```python
from build123d import *

# Parameters (mm, degrees)
EXTRUDE_1_DEPTH          = 7.5
CUT_EXTRUDE_1_DEPTH      = 30.546573405
CUT_EXTRUDE_1_DEPTH_BACK = 30.546573405
SKETCH_2_W               = 20
SKETCH_2_H               = 20
SKETCH_11_W              = 29.504788154
SKETCH_11_H              = 47.493911142
CUT_EXTRUDE_7_DEPTH      = 1
SKETCH_12_W              = 20.237973212
SKETCH_12_H              = 25.719397838
CUT_EXTRUDE_8_DEPTH      = 1
FILLET_1_R               = 5
FILLET_2_R               = 5
CUT_EXTRUDE_2_DEPTH      = 39.745967532
CUT_EXTRUDE_2_DEPTH_BACK = 39.745967532
SKETCH_3_R               = 4.2
CUT_EXTRUDE_3_DEPTH      = 39.745967532
CUT_EXTRUDE_3_DEPTH_BACK = 39.745967532
SKETCH_4_R               = 4.2
EXTRUDE_2_DEPTH          = 15
SKETCH_6_R               = 4.2
SKETCH_6_R_2             = 3.5
EXTRUDE_3_DEPTH          = 3.4
EXTRUDE_START            = -3.4
SKETCH_13_R              = 4.2
SKETCH_13_R_2            = 3.5
EXTRUDE_4_DEPTH          = 3.4
SKETCH_14_R              = 50
EXTRUDE_5_DEPTH          = 10
CUT_EXTRUDE_START        = -10
CUT_EXTRUDE_9_DEPTH      = 10
CHAMFER_1_SIZE           = 5
CUT_EXTRUDE_10_DEPTH     = 15
PATTERN_CIRCULAR_1_COUNT = 4


with BuildPart() as part:
    # ｽｹｯﾁ1 → ﾎﾞｽ - 押し出し1 (new, symmetric)
    with BuildSketch(Plane.XY):
        Polygon((7.455844123, -18), (18, -7.455844123), (18, 7.455844123), (7.455844123, 18), (-7.455844123, 18), (-18, 7.455844123), (-18, -7.455844123), (-7.455844123, -18), align=None)
    extrude(amount=EXTRUDE_1_DEPTH, both=True)

    # ｽｹｯﾁ2 → ｶｯﾄ - 押し出し1 (cut, two sides: drawn at the far end of the back side and taken through both)
    with BuildSketch(Plane.XY.offset(7.5).offset(-CUT_EXTRUDE_1_DEPTH_BACK)):
        Rectangle(SKETCH_2_W, SKETCH_2_H)
    extrude(amount=CUT_EXTRUDE_1_DEPTH + CUT_EXTRUDE_1_DEPTH_BACK, mode=Mode.SUBTRACT)

    # ｽｹｯﾁ11 → ｶｯﾄ - 押し出し7 (cut)
    with BuildSketch(Plane(origin=(0, 18, 0), x_dir=(1, 0, 0), z_dir=(0, 1, 0))):
        Rectangle(SKETCH_11_W, SKETCH_11_H)
    cut_extrude_7 = extrude(amount=-CUT_EXTRUDE_7_DEPTH, mode=Mode.SUBTRACT)

    # ﾐﾗｰ1: ｶｯﾄ - 押し出し7 across plane
    add(cut_extrude_7.mirror(Plane.ZX), mode=Mode.SUBTRACT)

    # ｽｹｯﾁ12 → ｶｯﾄ - 押し出し8 (cut)
    with BuildSketch(Plane.ZY.offset(18)):
        Rectangle(SKETCH_12_W, SKETCH_12_H)
    cut_extrude_8 = extrude(amount=-CUT_EXTRUDE_8_DEPTH, mode=Mode.SUBTRACT)

    # ﾐﾗｰ2: ｶｯﾄ - 押し出し8 across plane
    add(cut_extrude_8.mirror(Plane(origin=(0, 0, 0), x_dir=(0, 0, 1), z_dir=(1, 0, 0))), mode=Mode.SUBTRACT)

    # ﾌｨﾚｯﾄ1
    fillet_1_edges = [part.edges().sort_by_distance(p)[0] for p in [
        (-10, -10, 0),
        (-10, 10, 0),
        (10, 10, 0),
        (10, -10, 0),
    ]]
    fillet(fillet_1_edges, radius=FILLET_1_R)

    # ﾌｨﾚｯﾄ2
    fillet_2_edges = [part.edges().sort_by_distance(p)[0] for p in [
        (17, 8.455844123, 0),
        (17, -8.455844123, 0),
        (-8.455844123, 17, 0),
        (8.455844123, 17, 0),
        (8.455844123, -17, 0),
        (-8.455844123, -17, 0),
        (-17, -8.455844123, 0),
        (-17, 8.455844123, 0),
    ]]
    fillet(fillet_2_edges, radius=FILLET_2_R)

    # ｽｹｯﾁ3 → ｶｯﾄ - 押し出し2 (cut, two sides: drawn at the far end of the back side and taken through both)
    with BuildSketch(Plane.XZ.offset(17).offset(-CUT_EXTRUDE_2_DEPTH_BACK)):
        with Locations(Location((0, 0, 0), (0, 0, 270))):
            Circle(SKETCH_3_R)
    extrude(amount=CUT_EXTRUDE_2_DEPTH + CUT_EXTRUDE_2_DEPTH_BACK, mode=Mode.SUBTRACT)

    # ｽｹｯﾁ4 → ｶｯﾄ - 押し出し3 (cut, two sides: drawn at the far end of the back side and taken through both)
    with BuildSketch(Plane(origin=(17, 0, 0), x_dir=(0, 0, -1), z_dir=(1, 0, 0)).offset(-CUT_EXTRUDE_3_DEPTH_BACK)):
        Circle(SKETCH_4_R)
    extrude(amount=CUT_EXTRUDE_3_DEPTH + CUT_EXTRUDE_3_DEPTH_BACK, mode=Mode.SUBTRACT)

    # ｽｹｯﾁ5 → ﾎﾞｽ - 押し出し2 (add)
    with BuildSketch(Plane.XY.offset(7.5)):
        with BuildLine():
            Line((17, -6.384776311), (17, 6.384776311))
            ThreePointArc((17, 6.384776311), (16.619397663, 8.298193473), (15.535533906, 9.920310217))
            Line((15.535533906, 9.920310217), (9.920310217, 15.535533906))
            ThreePointArc((9.920310217, 15.535533906), (8.298193473, 16.619397663), (6.384776311, 17))
            Line((6.384776311, 17), (-6.384776311, 17))
            ThreePointArc((-6.384776311, 17), (-8.298193473, 16.619397663), (-9.920310217, 15.535533906))
            Line((-9.920310217, 15.535533906), (-15.535533906, 9.920310217))
            ThreePointArc((-15.535533906, 9.920310217), (-16.619397663, 8.298193473), (-17, 6.384776311))
            Line((-17, 6.384776311), (-17, -6.384776311))
            ThreePointArc((-17, -6.384776311), (-16.619397663, -8.298193473), (-15.535533906, -9.920310217))
            Line((-15.535533906, -9.920310217), (-9.920310217, -15.535533906))
            ThreePointArc((-9.920310217, -15.535533906), (-8.298193473, -16.619397663), (-6.384776311, -17))
            Line((-6.384776311, -17), (6.384776311, -17))
            ThreePointArc((6.384776311, -17), (8.298193473, -16.619397663), (9.920310217, -15.535533906))
            Line((9.920310217, -15.535533906), (15.535533906, -9.920310217))
            ThreePointArc((15.535533906, -9.920310217), (16.619397663, -8.298193473), (17, -6.384776311))
        make_face()
        with BuildLine():
            Line((5, 10), (-5, 10))
            ThreePointArc((-5, 10), (-8.535533906, 8.535533906), (-10, 5))
            Line((-10, 5), (-10, -5))
            ThreePointArc((-10, -5), (-8.535533906, -8.535533906), (-5, -10))
            Line((-5, -10), (5, -10))
            ThreePointArc((5, -10), (8.535533906, -8.535533906), (10, -5))
            Line((10, -5), (10, 5))
            ThreePointArc((10, 5), (8.535533906, 8.535533906), (5, 10))
        make_face(mode=Mode.SUBTRACT)
    extrude(amount=EXTRUDE_2_DEPTH)

    # ｽｹｯﾁ6 → ﾎﾞｽ - 押し出し3 (add)
    with BuildSketch(Plane.XZ.offset(17)):
        Circle(SKETCH_6_R)
        Circle(SKETCH_6_R_2, mode=Mode.SUBTRACT)
    extrude_3 = extrude(amount=-EXTRUDE_3_DEPTH)

    # ﾐﾗｰ3: ﾎﾞｽ - 押し出し3 across plane
    add(extrude_3.mirror(Plane.ZX))

    # ｽｹｯﾁ13 → ﾎﾞｽ - 押し出し4 (add)
    with BuildSketch(Plane.ZY.offset(17).offset(EXTRUDE_START)):
        Circle(SKETCH_13_R)
        Circle(SKETCH_13_R_2, mode=Mode.SUBTRACT)
    extrude_4 = extrude(amount=EXTRUDE_4_DEPTH)

    # ﾐﾗｰ4: ﾎﾞｽ - 押し出し4 across plane
    add(extrude_4.mirror(Plane(origin=(0, 0, 0), x_dir=(0, 0, 1), z_dir=(1, 0, 0))))

    # ｽｹｯﾁ14 → ﾎﾞｽ - 押し出し5 (add)
    with BuildSketch(Plane.XY.offset(22.5)):
        Circle(SKETCH_14_R)
        with BuildLine():
            Line((-5, -10), (5, -10))
            ThreePointArc((5, -10), (8.535533906, -8.535533906), (10, -5))
            Line((10, -5), (10, 5))
            ThreePointArc((10, 5), (8.535533906, 8.535533906), (5, 10))
            Line((5, 10), (-5, 10))
            ThreePointArc((-5, 10), (-8.535533906, 8.535533906), (-10, 5))
            Line((-10, 5), (-10, -5))
            ThreePointArc((-10, -5), (-8.535533906, -8.535533906), (-5, -10))
        make_face(mode=Mode.SUBTRACT)
    extrude(amount=EXTRUDE_5_DEPTH)

    # ｽｹｯﾁ15 → ｶｯﾄ - 押し出し9 (cut)
    with BuildSketch(Plane.XY.offset(32.5).offset(CUT_EXTRUDE_START)):
        with BuildLine():
            ThreePointArc((21.794494718, 45), (0, 50), (-21.794494718, 45))
            Line((-21.794494718, 45), (21.794494718, 45))
        make_face()
        with BuildLine():
            Line((45, 21.794494718), (45, -21.794494718))
            ThreePointArc((45, -21.794494718), (48.733971724, -11.180339887), (50, 0))
            ThreePointArc((50, 0), (48.733971724, 11.180339887), (45, 21.794494718))
        make_face()
        with BuildLine():
            Line((21.794494718, -45), (-21.794494718, -45))
            ThreePointArc((-21.794494718, -45), (0, -50), (21.794494718, -45))
        make_face()
        with BuildLine():
            ThreePointArc((-45, 21.794494718), (-50, 0), (-45, -21.794494718))
            Line((-45, -21.794494718), (-45, 21.794494718))
        make_face()
    extrude(amount=CUT_EXTRUDE_9_DEPTH, mode=Mode.SUBTRACT)

    # 面取り1
    chamfer_1_edges = [part.edges().sort_by_distance(p)[0] for p in [
        (16.619397663, -8.298193473, 22.5),
        (17, 0, 22.5),
        (16.619397663, 8.298193473, 22.5),
        (12.727922061, 12.727922061, 22.5),
        (8.298193473, 16.619397663, 22.5),
        (0, 17, 22.5),
        (-8.298193473, 16.619397663, 22.5),
        (-12.727922061, 12.727922061, 22.5),
        (-16.619397663, 8.298193473, 22.5),
        (-17, 0, 22.5),
        (-16.619397663, -8.298193473, 22.5),
        (-12.727922061, -12.727922061, 22.5),
        (-8.298193473, -16.619397663, 22.5),
        (0, -17, 22.5),
        (8.298193473, -16.619397663, 22.5),
        (12.727922061, -12.727922061, 22.5),
    ]]
    chamfer(chamfer_1_edges, length=CHAMFER_1_SIZE)

    # ｽｹｯﾁ16 → ｶｯﾄ - 押し出し10 (cut)
    with BuildSketch(Plane.ZY.offset(45)):
        Polygon((28.8, 12.5), (28.15, 13.625833025), (26.85, 13.625833025), (26.2, 12.5), (26.85, 11.374166975), (28.15, 11.374166975), align=None)
        Polygon((28.8, -12.5), (28.15, -11.374166975), (26.85, -11.374166975), (26.2, -12.5), (26.85, -13.625833025), (28.15, -13.625833025), align=None)
    cut_extrude_10 = extrude(amount=-CUT_EXTRUDE_10_DEPTH, mode=Mode.SUBTRACT)

    # 円形ﾊﾟﾀｰﾝ1: ｶｯﾄ - 押し出し10 ×4 about axis
    pattern_circular_1_axis = Axis((0, 0, 0), (0, 0, 1))
    for i in range(1, PATTERN_CIRCULAR_1_COUNT):
        add(cut_extrude_10.rotate(pattern_circular_1_axis, i * 360 / PATTERN_CIRCULAR_1_COUNT), mode=Mode.SUBTRACT)


solid = part.part
```
The listing builds one solid part. Answer for the finished solid, in the listing's coordinates (mm). A direction names the side the tool comes from. Coordinates: 2 decimals unless noted, no trailing zeros. Loops run counter-clockwise (first coordinate to the right, second up) from the corner with the lowest first, then second, coordinate; pieces in that order, holes last. Notation, with made-up numbers: (41.5, -35.5) -> (67.5, -35.5) arc R18 cw to (67.5, -18.5) -> close; hole circle Ø5 at (86, 83.25). An arc over 180 degrees is marked (long way). Return JSON: item names as keys, results as strings. Group by question number.
(1) A cutting plane is placed at A-A on x = 0. Count the separate pieces of the cut face and the enclosed holes in it, and give its area (3 significant figures).
(2) Find the intervals of material crossed by probe 1 along Y at (x, z) = (-3.5, 13); probe 2 along X at (y, z) = (-35, 27.5); probe 3 along Z at (x, y) = (0, 15.9), in increasing order. Write a range as from..to.
(3) Given pin 1 Ø1.4 at (y, z) = (38.5, 27.5) entering from -X; pin 2 Ø1 at (x, z) = (4, 5) entering from +Y; pin 3 Ø12 at (y, z) = (32, 27) entering from -X, each flat-ended and moving along its own axis, determine where each tip first touches the part or whether it passes through.
(4) Which of the six approach directions +Z, -Z, +X, -X, +Y, -Y give full straight-line access (tool end or side, diameter ignored) to faces 5 (the flat face through (-12.767, -12.689, 4.825)), 6 (the flat face through (12.767, 12.689, 4.825)), 7 (the flat face through (17, 0, 5)), 8 (the flat face through (-12.689, 12.767, 4.825)), 9 (the flat face through (0, 17, 5))?
(5) Determine the mould class of faces 1 (the flat face through (19, -19, 22.5)), 2 (the cylindrical face through (8, -9, 12)), 3 (the cylindrical face through (-9, -8, 12)), 4 (the conical face through (18.91, 9.2, 19.96)) for opening direction Y: released by +Y, released by -Y, zero draft, split by the parting line, or undercut.
(6) A cutting plane is placed at C-C on z = 25. Write down the section's boundary in (x, y), and give its area (3 significant figures).
The answers:
{
 "1": {"separate pieces": "4", "enclosed holes": "0", "area": "1,040 mm^2"},
 "2": {"probe 1": "y = -17..-10, 10..17", "probe 2": "x = -35.71..-13.63, -11.37..11.37, 13.63..35.71", "probe 3": "z = -7.5..-3.5, 3.5..32.5"},
 "3": {"pin 1": "stops at x = -32.73", "pin 2": "stops at y = 17", "pin 3": "stops at x = -42.71"},
 "4": {"face 5": "-Z, -X, -Y", "face 6": "-Z, +X, +Y", "face 7": "-Z, +X, +Y, -Y", "face 8": "-Z, -X, +Y", "face 9": "-Z, +X, -X, +Y"},
 "5": {"face 1": "zero draft", "face 2": "undercut", "face 3": "undercut", "face 4": "released by +Y"},
 "6": {"outline": "(-45, -21.79) arc R50 ccw to (-21.79, -45) -> (21.79, -45) arc R50 ccw to (45, -21.79) -> (45, 21.79) arc R50 ccw to (21.79, 45) -> (-21.79, 45) arc R50 ccw to (-45, 21.79) -> close; hole (-10, -5) arc R5 ccw to (-5, -10) -> (5, -10) arc R5 ccw to (10, -5) -> (10, 5) arc R5 ccw to (5, 10) -> (-5, 10) arc R5 ccw to (-10, 5) -> close", "area": "6,890 mm^2"}
}
